Build history of the part. All positions in model axes, mm. Face numbers are marked on the shaded views. Give positions to 0.01 mm unless a question says otherwise; leave off trailing zeros. Write each loop counter-clockwise with the first axis right and the second up, starting at its lowest first coordinate (ties: lowest second). Pieces come first, ordered by that corner, then holes.
from build123d import *

# Parameters (mm, degrees)
BOSS_EXTRUDE1_DEPTH = 3
SKETCH4_R           = 1.65
CUT_EXTRUDE1_DEPTH  = 4


with BuildPart() as part:
    # Sketch5 → Boss-Extrude1 (new body)
    with BuildSketch(Plane(origin=(0, 0, 0), x_dir=(0, 1, 0), z_dir=(0, 0, 1))):
        with BuildLine():
            ThreePointArc((37.723245901, 9.079766174), (42.363354518, 14.24854402), (43.948073482, 21.011349518))
            ThreePointArc((43.948073482, 21.011349518), (49.906664226, 28.911044217), (58.985716635, 24.976481046))
            ThreePointArc((58.985716635, 24.976481046), (60.156028849, 23.886109344), (61.747774642, 23.728354912))
            ThreePointArc((61.747774642, 23.728354912), (49.889938389, 43.437501627), (32.000159984, 57.894837948))
            ThreePointArc((32.000159984, 57.894837948), (31.906399176, 56.411758551), (32.670933348, 55.137473226))
            ThreePointArc((32.670933348, 55.137473226), (36.27043514, 43.073301984), (27.113180378, 34.433549317))
            ThreePointArc((27.113180378, 34.433549317), (21.388023687, 31.800064681), (17.397863538, 26.922433858))
            ThreePointArc((17.397863538, 26.922433858), (17.377786203, 26.87598895), (17.362505758, 26.82775269))
            ThreePointArc((17.362505758, 26.82775269), (22.00306193, 11.670310925), (37.63394302, 9.032440796))
            ThreePointArc((37.63394302, 9.032440796), (37.679793297, 9.053841282), (37.723245901, 9.079766174))
        make_face()
    extrude(amount=BOSS_EXTRUDE1_DEPTH)

    # Sketch4 → Cut-Extrude1 (cut, through all)
    with BuildSketch(Plane(origin=(0, 0, 0), x_dir=(0, 1, 0), z_dir=(0, 0, 1))):
        with Locations((40.305086528, 40.305086528)):
            Circle(SKETCH4_R)
        with Locations((46.691666524, 32.693856872)):
            Circle(SKETCH4_R)
    extrude(amount=CUT_EXTRUDE1_DEPTH, mode=Mode.SUBTRACT)


solid = part.part
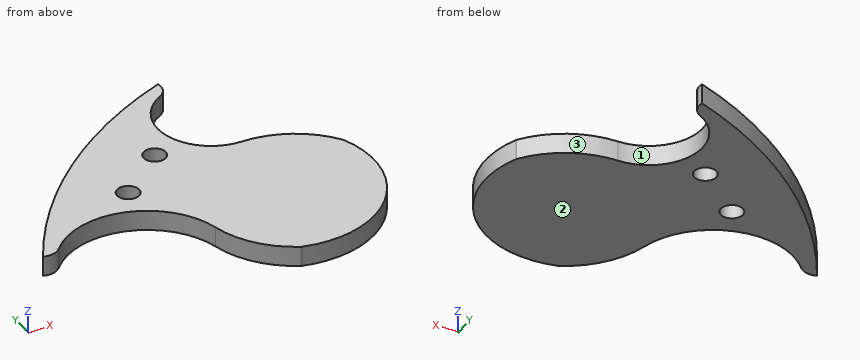
(1) Saw through at C-C, the plane x = -13. List the corners of the cut face in (y, z), plus the area to 3 significant figures.
(2) Saw through at D-D, the plane y = 23. List the corners of the cut face in (x, z), plus the area to 3 significant figures.
(3) Probe line 1 (Y direction, x = -31.5, z = 0.4); line 2 (X direction, y = 40, z = 2.85); line 3 (Y direction, x = -33.5, z = 2.95). List the from-to ranges inside material, lowest first.
(4) Saw through at A-A, the plane y = 40.5. List the corners of the cut face in (x, z), plus the area to 3 significant figures.
(5) Drop flat-ended pins along their axis: pin 1 (1.5 mm diameter, centred on x = -47, z = 2.5, fed in from -Y); pin 2 (1 mm diameter, centred on x = -16, z = 2, fed in from +Y); pin 3 (1.5 mm diameter, centred on x = -50.5, z = 1.5, fed in from +Y). Give the stop position or say it passes through.
(6) Saw through at B-B, the plane z = 1. List the corners of the cut face in (x, y).
(7) Mould opens along Y. For the marked faces 1, 2 and 3 say: +Y half, -Y half, draft (parallel to the pull), parting line (faces both ways), or undercut.
Computed values:
1. outline: (20.67, 0) - (41.63, 0) - (41.63, 3) - (20.67, 3) - close
1. area: 62.9 mm2
2. outline: (-32.88, 0) - (-10.87, 0) - (-10.87, 3) - (-32.88, 3) - close
2. area: 66.0 mm2
3. line 1: y = 21.01 to 45.55, 47.83 to 58.17
3. line 2: x = -52.69 to -41.93, -38.68 to -10.98
3. line 3: y = 24.23 to 45.25, 48.13 to 57.04
4. outline: (-52.3, 0) - (-41.94, 0) - (-41.94, 3) - (-52.3, 3) - close; (-38.67, 0) - (-11.52, 0) - (-11.52, 3) - (-38.67, 3) - close
4. area: 113 mm2
5. pin 1: stops at y = 36.58
5. pin 2: stops at y = 43.3
5. pin 3: stops at y = 43.6
6. outline: (-57.89, 32) arc R2.5 ccw to (-55.14, 32.67) arc R12 cw to (-34.43, 27.11) arc R14 ccw to (-26.92, 17.4) arc R0.5 ccw to (-26.83, 17.36) arc R15.08 ccw to (-9.03, 37.63) arc R0.5 ccw to (-9.08, 37.72) arc R14 ccw to (-21.01, 43.95) arc R8 cw to (-24.98, 58.99) arc R2.5 ccw to (-23.73, 61.75) arc R66.15 ccw to start; hole circle Ø3.3 at (-40.31, 40.31); hole circle Ø3.3 at (-32.69, 46.69)
7. face 1: undercut
7. face 2: draft
7. face 3: +Y half
